from build123d import *

# Parameters (mm, degrees)
SKETCH1_W           = 52
SKETCH1_H           = 24
SKETCH1_R           = 4
SKETCH1_R_2         = 1.5
BOSS_EXTRUDE1_DEPTH = 2
SKETCH3_R           = 4
SKETCH3_R_2         = 1.5
BOSS_EXTRUDE2_DEPTH = 2
FILLET1_R           = 2
FILLET2_R           = 1
BOSS_EXTRUDE3_START = 2
SKETCH5_R           = 4
SKETCH5_R_2         = 1.5
BOSS_EXTRUDE3_DEPTH = 2
FILLET3_R           = 2
FILLET4_R           = 1


with BuildPart() as part:
    # Sketch1 → Boss-Extrude1 (new body)
    with BuildSketch(Plane(origin=(0, 0, 0), x_dir=(1, 0, 0), z_dir=(0, 1, 0))):
        Rectangle(SKETCH1_W, SKETCH1_H)
        with Locations(Location((0, 0, 0), (0, 0, 270))):
            Circle(SKETCH1_R, mode=Mode.SUBTRACT)
        with Locations(Location((0, 7, 0), (0, 0, 270))):
            Circle(SKETCH1_R_2, mode=Mode.SUBTRACT)
        with Locations(Location((0, -7, 0), (0, 0, 270))):
            Circle(SKETCH1_R_2, mode=Mode.SUBTRACT)
        with Locations(Location((7, 0, 0), (0, 0, 270))):
            Circle(SKETCH1_R_2, mode=Mode.SUBTRACT)
        with Locations(Location((-7, 0, 0), (0, 0, 270))):
            Circle(SKETCH1_R_2, mode=Mode.SUBTRACT)
        with Locations(Location((-15.5, 0, 0), (0, 0, 270))):
            Circle(SKETCH1_R_2, mode=Mode.SUBTRACT)
        with Locations(Location((15.5, 0, 0), (0, 0, 270))):
            Circle(SKETCH1_R_2, mode=Mode.SUBTRACT)
    extrude(amount=BOSS_EXTRUDE1_DEPTH)

    # Sketch3 → Boss-Extrude2 (add)
    with BuildSketch(Plane(origin=(26, 0, 0), x_dir=(0, 0, -1), z_dir=(1, 0, 0))):
        with BuildLine():
            Line((-12, 0), (12, 0))
            Line((12, 0), (12, 50))
            ThreePointArc((12, 50), (0, 62), (-12, 50))
            Line((-12, 50), (-12, 0))
        make_face()
        with Locations((0, 50)):
            Circle(SKETCH3_R, mode=Mode.SUBTRACT)
        with Locations((0, 57)):
            Circle(SKETCH3_R_2, mode=Mode.SUBTRACT)
        with Locations((7, 50)):
            Circle(SKETCH3_R_2, mode=Mode.SUBTRACT)
        with Locations((0, 43)):
            Circle(SKETCH3_R_2, mode=Mode.SUBTRACT)
        with Locations((-7, 50)):
            Circle(SKETCH3_R_2, mode=Mode.SUBTRACT)
        with Locations((0, 31)):
            Circle(SKETCH3_R_2, mode=Mode.SUBTRACT)
        with Locations((0, 14)):
            Circle(SKETCH3_R_2, mode=Mode.SUBTRACT)
    extrude(amount=BOSS_EXTRUDE2_DEPTH)

    # Fillet1
    fillet1_edges = [part.edges().sort_by_distance(p)[0] for p in [
        (28, 0, 0),
    ]]
    fillet(fillet1_edges, radius=FILLET1_R)

    # Fillet2
    fillet2_edges = [part.edges().sort_by_distance(p)[0] for p in [
        (26, 2, 0),
    ]]
    fillet(fillet2_edges, radius=FILLET2_R)

    # Sketch5 → Boss-Extrude3 (add)
    with BuildSketch(Plane.ZY.offset(26).offset(BOSS_EXTRUDE3_START)):
        with BuildLine():
            Line((-12, 0), (-12, 50))
            ThreePointArc((-12, 50), (0, 62), (12, 50))
            Line((12, 50), (12, 0))
            Line((12, 0), (-12, 0))
        make_face()
        with Locations(Location((0, 50, 0), (0, 0, 180))):
            Circle(SKETCH5_R, mode=Mode.SUBTRACT)
        with Locations(Location((0, 57, 0), (0, 0, 180))):
            Circle(SKETCH5_R_2, mode=Mode.SUBTRACT)
        with Locations(Location((0, 43, 0), (0, 0, 180))):
            Circle(SKETCH5_R_2, mode=Mode.SUBTRACT)
        with Locations(Location((7, 50, 0), (0, 0, 180))):
            Circle(SKETCH5_R_2, mode=Mode.SUBTRACT)
        with Locations(Location((-7, 50, 0), (0, 0, 180))):
            Circle(SKETCH5_R_2, mode=Mode.SUBTRACT)
        with Locations(Location((0, 31, 0), (0, 0, 180))):
            Circle(SKETCH5_R_2, mode=Mode.SUBTRACT)
        with Locations(Location((0, 14, 0), (0, 0, 180))):
            Circle(SKETCH5_R_2, mode=Mode.SUBTRACT)
    extrude(amount=-BOSS_EXTRUDE3_DEPTH)

    # Fillet3
    fillet3_edges = [part.edges().sort_by_distance(p)[0] for p in [
        (-28, 0, 0),
    ]]
    fillet(fillet3_edges, radius=FILLET3_R)

    # Fillet4
    fillet4_edges = [part.edges().sort_by_distance(p)[0] for p in [
        (-26, 2, 0),
    ]]
    fillet(fillet4_edges, radius=FILLET4_R)


solid = part.part
Read the model definition and answer for the solid it produces. Units are mm, in the model's axes. A direction names the side the tool comes from. Coordinates: 2 decimals unless noted, no trailing zeros. Write each loop counter-clockwise with the first axis right and the second up, starting at its lowest first coordinate (ties: lowest second). Pieces come first, ordered by that corner, then holes. Notation, with made-up numbers: M 31,38 L 81,38 A15 cw 81,66 Z; hole C 45,-22.5 d2. An arc over 180 degrees is marked long. Use a Markdown table: item, result.
Q1. Which of the six approach directions +Z, -Z, +X, -X, +Y, -Y give full straight-line access (tool end or side, diameter ignored) to faces 4 (the face through (0, 0, -5)), 5 (the face through (0, 2, 5))?
Answer block:
| item | result |
|---|---|
| face 4 | +Z, -Z, +X, -X, -Y |
| face 5 | +Z, -Z, +Y |
Q2. Determine the mould class of faces 1 (the face through (27.4, 0.57, -0.17)), 2 (the face through (-15.05, 0.99, 1.43)), 3 (the face through (0, 1, 12)) for opening direction Z: released by +Z, released by -Z, zero draft, split by the parting line, or undercut.
Answer block:
| item | result |
|---|---|
| face 1 | zero draft |
| face 2 | undercut |
| face 3 | released by +Z |
Q3. The part is cut by section B-B, the plane x = -15.5. Write down the section's boundary in (y, z), then the cut area to 3 significant figures.
Answer block:
| item | result |
|---|---|
| outline | M 0,-12 L 2,-12 L 2,-1.5 L 0,-1.5 Z; M 0,1.5 L 2,1.5 L 2,12 L 0,12 Z |
| area | 42.0 mm2 |
Q4. The part is cut by section A-A, the plane y = 34. Write down the section's boundary in (x, z).
Answer block:
| item | result |
|---|---|
| outline | M -28,-12 L -26,-12 L -26,12 L -28,12 Z; M 26,-12 L 28,-12 L 28,12 L 26,12 Z |
Q5. The part is cut by section C-C, the plane y = 53. Write down the section's boundary in (x, z), then the cut area to 3 significant figures.
Answer block:
| item | result |
|---|---|
| outline | M -28,-11.62 L -26,-11.62 L -26,-2.65 L -28,-2.65 Z; M -28,2.65 L -26,2.65 L -26,11.62 L -28,11.62 Z; M 26,-11.62 L 28,-11.62 L 28,-2.65 L 26,-2.65 Z; M 26,2.65 L 28,2.65 L 28,11.62 L 26,11.62 Z |
| area | 71.8 mm2 |
Q6. Straight lines are drawn through the part: L1, parallel to X at y = 25, z = 4.5; L2, parallel to Y at x = 27.6, z = 0; L3, parallel to Y at x = -27.5, z = 0. For each, find the intervals that lie inside material, in ascending order. Write a range as [from, to].
Answer block:
| item | result |
|---|---|
| L1 | x = [-28, -26], [26, 28] |
| L2 | y = [0.8, 12.5], [15.5, 29.5], [32.5, 41.5], [44.5, 46], [54, 55.5], [58.5, 62] |
| L3 | y = [0.68, 12.5], [15.5, 29.5], [32.5, 41.5], [44.5, 46], [54, 55.5], [58.5, 62] |
Q7. Each of these flat-tipped pins is pushed along its axis until it touches: pin 1 Ø6 at (x, z) = (7, -6.5) entering from +Y; pin 2 Ø2.5 at (y, z) = (57, 0) entering from -X; pin 3 Ø4 at (y, z) = (50, 7) entering from -X. Where does it stop, or does it pass through?
Answer block:
| item | result |
|---|---|
| pin 1 | stops at y = 2 |
| pin 2 | passes through |
| pin 3 | stops at x = -28 |
Q8. The part is cut by section D-D, the plane z = 7. Write down the section's boundary in (x, y), then the cut area to 3 significant figures.
Answer block:
| item | result |
|---|---|
| outline | M -28,2 A2 ccw -26,0 L -1.5,0 L -1.5,2 L -25,2 A1 cw -26,3 L -26,48.5 L -28,48.5 Z; M -28,51.5 L -26,51.5 L -26,59.75 L -28,59.75 Z; M 1.5,0 L 26,0 A2 ccw 28,2 L 28,48.5 L 26,48.5 L 26,3 A1 cw 25,2 L 1.5,2 Z; M 26,51.5 L 28,51.5 L 28,59.75 L 26,59.75 Z |
| area | 324 mm2 |
